```python
from build123d import *

# Parameters (mm, degrees)
SKETCH_1_R          = 7.5
EXTRUDE_1_DEPTH     = 10
SKETCH_1_3_W        = 20
SKETCH_1_3_H        = 5
EXTRUDE_2_DEPTH     = 5
SKETCH_1_4_R        = 7.5
CUT_EXTRUDE_1_DEPTH = 5


with BuildPart() as part:
    # Sketch 1 → Extrude 1 (new body)
    with BuildSketch(Plane.XY):
        with BuildLine():
            Line((-7, 10), (7, 10))
            ThreePointArc((7, 10), (9.121320344, 9.121320344), (10, 7))
            Line((10, 7), (10, -17.5))
            Line((10, -17.5), (-10, -17.5))
            Line((-10, -17.5), (-10, 7))
            ThreePointArc((-10, 7), (-9.121320344, 9.121320344), (-7, 10))
        make_face()
        Circle(SKETCH_1_R, mode=Mode.SUBTRACT)
        Circle(SKETCH_1_R)
    extrude(amount=EXTRUDE_1_DEPTH)

    # Sketch 1_3 → Extrude 2 (add)
    with BuildSketch(Plane.XY):
        with Locations((0, -20)):
            Rectangle(SKETCH_1_3_W, SKETCH_1_3_H)
    extrude(amount=EXTRUDE_2_DEPTH)

    # Sketch 1_4 → Cut-Extrude 1 (cut)
    with BuildSketch(Plane.XY):
        Circle(SKETCH_1_4_R)
    extrude(amount=CUT_EXTRUDE_1_DEPTH, mode=Mode.SUBTRACT)


solid = part.part
```
Read the model definition and answer for the solid it produces. Units are mm, in the model's axes. A direction names the side the tool comes from. Give positions to 0.01 mm unless a question says otherwise; leave off trailing zeros. Write each loop counter-clockwise with the first axis right and the second up, starting at its lowest first coordinate (ties: lowest second). Pieces come first, ordered by that corner, then holes. Notation, with made-up numbers: (10.25, 78) -> (28.25, 78) arc R30 cw to (28.25, 116) -> close; hole circle Ø9 at (-10.75, 19.5). An arc over 180 degrees is marked (long way). Answer in a Markdown table with one row per item.
1) A tool of negligible diameter and unlimited length cuts with its end or side. For faces 1 (the flat face through (0, -10, 0)), 2 (the flat face through (0, -17.5, 7)), from which of +Z, -Z, +X, -X, +Y, -Y can it reach the whole face along a straight path? Write none if from no direction.
Results list:
| item | result |
|---|---|
| face 1 | -Z, +X, -X, +Y, -Y |
| face 2 | +Z, +X, -X, -Y |
2) Section B-B on z = 7.5 is taken. Give the vertices of the cut face in (x, y), plus the area to 3 significant figures.
Results list:
| item | result |
|---|---|
| outline | (-10, -17.5) -> (10, -17.5) -> (10, 7) arc R3 ccw to (7, 10) -> (-7, 10) arc R3 ccw to (-10, 7) -> close |
| area | 546 mm^2 |
3) Straight lines are drawn through the part: line 1 (Y direction, x = 0, z = 1.2); line 2 (Z direction, x = 5, y = 3); line 3 (Y direction, x = 3.75, z = 5.5). For each, find the intervals that lie inside material, in ascending order. Write a range as [from, to].
Results list:
| item | result |
|---|---|
| line 1 | [-22.5, -7.5], [7.5, 10] |
| line 2 | [5, 10] |
| line 3 | [-17.5, 10] |
4) Determine the mould class of faces 3 (the flat face through (0, -20, 5)), 4 (the flat face through (10, -8, 5)), 5 (the cylindrical face through (-7.493, 0.33, 2.465)), 6 (the flat face through (0, 0, 5)) for opening direction X: released by +X, released by -X, zero draft, split by the parting line, or undercut.
Results list:
| item | result |
|---|---|
| face 3 | zero draft |
| face 4 | released by +X |
| face 5 | undercut |
| face 6 | undercut |
5) Section D-D on x = 0.5 is taken. Give the vertices of the cut face in (y, z).
Results list:
| item | result |
|---|---|
| outline | (-22.5, 0) -> (-7.48, 0) -> (-7.48, 5) -> (7.48, 5) -> (7.48, 0) -> (10, 0) -> (10, 10) -> (-17.5, 10) -> (-17.5, 5) -> (-22.5, 5) -> close |
6) Section A-A on x = -6.5 is taken. Give the vertices of the cut face in (y, z), plus the area to 3 significant figures.
Results list:
| item | result |
|---|---|
| outline | (-22.5, 0) -> (-3.74, 0) -> (-3.74, 5) -> (3.74, 5) -> (3.74, 0) -> (10, 0) -> (10, 10) -> (-17.5, 10) -> (-17.5, 5) -> (-22.5, 5) -> close |
| area | 263 mm^2 |
7) Each of these flat-tipped pins is pushed along its axis until it touches: pin 1 Ø1.5 at (x, y) = (1, -21) entering from +Z; pin 2 Ø7.5 at (x, y) = (-1, -0.5) entering from -Z. Where does it stop, or does it pass through?
Results list:
| item | result |
|---|---|
| pin 1 | z = 5 |
| pin 2 | z = 5 |
8) Section C-C on y = 0 is taken. Give the vertices of the cut face in (x, z), plus the area to 3 significant figures.
Results list:
| item | result |
|---|---|
| outline | (-10, 0) -> (-7.5, 0) -> (-7.5, 5) -> (7.5, 5) -> (7.5, 0) -> (10, 0) -> (10, 10) -> (-10, 10) -> close |
| area | 125 mm^2 |
